Here's how the part is built. I have some questions about the finished solid (model axes, mm). A direction names the side the tool comes from. Round coordinates to 2 decimals unless told otherwise and drop trailing zeros. Loops run counter-clockwise (first coordinate to the right, second up) from the corner with the lowest first, then second, coordinate; pieces in that order, holes last. Notation, with made-up numbers: M 37.25,76.25 L 91.25,76.25 A31 cw 91.25,107.25 Z; hole C 69.25,66.25 d11. An arc over 180 degrees is marked long. Answer as a JSON object with one key per item and string values.
from build123d import *

# Parameters (mm, degrees)
F1_DEPTH      = 20
F2_R          = 15
F3_DEPTH      = 5
F3_DEPTH_BACK = 55
F4_W          = 15
F4_H          = 20
F5_DEPTH      = 25
F6_R          = 9.99999
F7_W          = 15
F7_H          = 10
F8_DEPTH      = 25
F9_DEPTH      = 25
F10_DEPTH     = 5


# Not quite as in the source:
# - a fillet or chamfer is up to 0.001 mm smaller than in the source, because OpenCascade refuses the exact size


with BuildPart() as f1:
    # F0 (on Front) → F1 (new body)
    with BuildSketch(Plane.XZ):
        with BuildLine():
            ThreePointArc((18.649535318, 7.2245991185), (19.659485069, 3.6748669119), (20, 0))
            ThreePointArc((20, 0), (0, -20), (-20, 0))
            Line((-20, 0), (-20, -50))
            Line((-20, -50), (-5, -50))
            Line((-5, -50), (-5, -30))
            Line((-5, -30), (15, -30))
            Line((15, -30), (15, -80))
            Line((15, -80), (30, -80))
            Line((30, -80), (30, -22.0754199539))
            Line((30, -22.0754199539), (18.649535318, 7.2245991185))
        make_face()
        with BuildLine():
            ThreePointArc((-20, 0), (0, -20), (20, 0))
            ThreePointArc((20, 0), (19.659485069, 3.6748669119), (18.649535318, 7.2245991185))
            ThreePointArc((18.649535318, 7.2245991185), (-3.6748669119, 19.659485069), (-20, 0))
        make_face()
    extrude(amount=-F1_DEPTH)

    # F2 (on face) → F3 (join, two sides)
    with BuildSketch(Plane.XZ) as f3_sk:
        Circle(F2_R)
    extrude(amount=F3_DEPTH)
    extrude(f3_sk.sketch, amount=-F3_DEPTH_BACK)

    # F4 (on face) → F5 (join)
    with BuildSketch(Plane.XZ):
        with Locations((22.5, -70)):
            Rectangle(F4_W, F4_H)
    extrude(amount=F5_DEPTH)

    # F6 (radius 10 in the source; OpenCascade refuses exactly that, so slightly less here)
    f6_edges = [f1.edges().sort_by_distance(p)[0] for p in [
        (22.5, -25, -60),
        (22.5, -25, -80),
    ]]
    fillet(f6_edges, radius=F6_R)

    # F7 (on face) → F8 (join)
    with BuildSketch(Plane(origin=(0, 55, 0), x_dir=(-1, 0, 0), z_dir=(0, 1, 0))):
        with Locations((37.5, 10)):
            Rectangle(F7_W, F7_H)
        with BuildLine():
            Line((30, 15), (0, 15))
            ThreePointArc((0, 15), (10.6066017178, 10.6066017178), (15, 0))
            ThreePointArc((15, 0), (10.6066017178, -10.6066017178), (0, -15))
            Line((0, -15), (45, -15))
            Line((45, -15), (45, 5))
            Line((45, 5), (30, 5))
            Line((30, 5), (30, 15))
        make_face()
    extrude(amount=-F8_DEPTH)

    # F7 (on face) → F9 (cut)
    with BuildSketch(Plane(origin=(0, 55, 0), x_dir=(-1, 0, 0), z_dir=(0, 1, 0))):
        with Locations((37.5, 10)):
            Rectangle(F7_W, F7_H)
    extrude(amount=-F9_DEPTH, mode=Mode.SUBTRACT)

    # F7 (on face) → F10 (cut)
    with BuildSketch(Plane(origin=(0, 55, 0), x_dir=(-1, 0, 0), z_dir=(0, 1, 0))):
        with Locations((37.5, 10)):
            Rectangle(F7_W, F7_H)
        with BuildLine():
            Line((30, 15), (0, 15))
            ThreePointArc((0, 15), (10.6066017178, 10.6066017178), (15, 0))
            ThreePointArc((15, 0), (10.6066017178, -10.6066017178), (0, -15))
            Line((0, -15), (45, -15))
            Line((45, -15), (45, 5))
            Line((45, 5), (30, 5))
            Line((30, 5), (30, 15))
        make_face()
    extrude(amount=-F10_DEPTH, mode=Mode.SUBTRACT)


solid = f1.part
Item 1: For faces 1 (the face through (-20, 10, -25)), 2 (the face through (-22, 40, -15)), 3 (the face through (-13, 10, -50)), 4 (the face through (-15, 40, 15)), which set-ups out of +Z, -Z, +X, -X, +Y, -Y let a thin tool reach every point of the face, with its end or its side?
Solution:
{"face 1": "+Z, -Z, -X, -Y", "face 2": "-Z, +X, -X, +Y", "face 3": "-Z, -X, +Y, -Y", "face 4": "+Z, +X, -X, +Y"}
Item 2: For P1, Ø4, axis at x = 21.5, z = -4.5, coming from the -Y side; P2, Ø7.5, axis at x = 23, y = -4, coming from the +Z side; P3, Ø16.5, axis at x = -34.5, y = 36, coming from the +Z side; P4, Ø12, axis at y = 21, z = -40, coming from the +X side, each with a flat end and sliding along its axis, tell me the tip position at first contact or that it passes through.
Solution:
{"P1": "stops at y = 0", "P2": "stops at z = -60", "P3": "stops at z = 15", "P4": "stops at x = 30"}
Item 3: I want a section at A-A on z = -44. List the corners of the cut face in (x, y) for me.
Solution:
{"outline": "M -20,0 L -5,0 L -5,20 L -20,20 Z; M 15,0 L 30,0 L 30,20 L 15,20 Z"}
Item 4: I want a section at B-B on y = 2. List the corners of the cut face in (x, z) for me.
Solution:
{"outline": "M -20,-50 L -5,-50 L -5,-30 L 15,-30 L 15,-80 L 30,-80 L 30,-22.08 L 18.65,7.22 A20 ccw -20,0 Z"}
Item 5: If I drill on L1, parallel to Y at x = 15, z = 2; L2, parallel to Z at x = -24.5, y = 44.5; L3, parallel to Y at x = 10.5, z = 5.5, over which ranges is the centre line in solid material (lowest first)? Write a range as from..to.
Solution:
{"L1": "y = 0..20", "L2": "z = -15..15", "L3": "y = -5..55"}
Item 6: I want a section at D-D on z = -62. List the corners of the cut face in (x, y) for me.
Solution:
{"outline": "M 15,-21 L 30,-21 L 30,20 L 15,20 Z"}
Item 7: We'd pull the mould along Y, two halves only. Please class faces 5 (the face through (15, 3, -61)), 6 (the face through (13.856, 37.255, -5.745)), 7 (the face through (5, 0, -19)): +Y half, -Y half, draft (parallel to the pull), parting line (faces both ways), or undercut.
Solution:
{"face 5": "draft", "face 6": "undercut", "face 7": "-Y half"}
Item 8: I want a section at C-C on x = 7. List the corners of the cut face in (y, z) for me (1 decimal), plus the area to 3 significant figures.
Solution:
{"outline": "M -5,-13.3 L 0,-13.3 L 0,-30 L 20,-30 L 20,-13.3 L 55,-13.3 L 55,13.3 L 20,13.3 L 20,18.7 L 0,18.7 L 0,13.3 L -5,13.3 Z", "area": "2,040 mm2"}
